Build history of the part. All positions in model axes, mm. Face numbers are marked on the shaded views. A direction names the side the tool comes from. Give positions to 0.01 mm unless a question says otherwise; leave off trailing zeros. Loops run counter-clockwise (first coordinate to the right, second up) from the corner with the lowest first, then second, coordinate; pieces in that order, holes last. Notation, with made-up numbers: (66.25, 15) - (79.25, 15) arc R6 cw to (79.25, 24) - close; hole circle Ø10 at (5.5, -30). An arc over 180 degrees is marked (long way). Return JSON: item names as keys, results as strings. Group by question number.
1) Drop flat-ended pins along their axis: pin 1 (4 mm diameter, centred on x = -3.5, y = 48, fed in from -Z); pin 2 (19 mm diameter, centred on y = 18.5, z = 6.5, fed in from -X); pin 3 (8 mm diameter, centred on x = 29.5, z = 0.5, fed in from -Y). Give the stop position or say it passes through.
2) Slice it at B-B (y = -7). List the corners of the cut face in (x, z), and give its area (3 significant figures).
3) Mould opens along Z. For the marked faces 6, 7 and 8 say: released by +Z, released by -Z, zero draft, split by the parting line, or undercut.
4) Slice it at C-C (x = 12.5). List the corners of the cut face in (y, z).
5) Slice it at D-D (y = 34). List the corners of the cut face in (x, z).
6) 3-axis set-ups, long thin cutter, end or side, ignore diameter. For the marked faces 1, 2, 3, 4 and 5: which of +Z, -Z, +X, -X, +Y, -Y reach the whole face in a straight line?
7) Drill centre lines: probe 1 along Y at (x, z) = (-7, 0); probe 2 along Z at (x, y) = (4.5, 10.5); probe 3 along X at (y, z) = (49, 19). Where is each one in solid material? Low to high. Write a range as from..to.
8) Slice it at A-A (z = 10). List the corners of the cut face in (x, y).
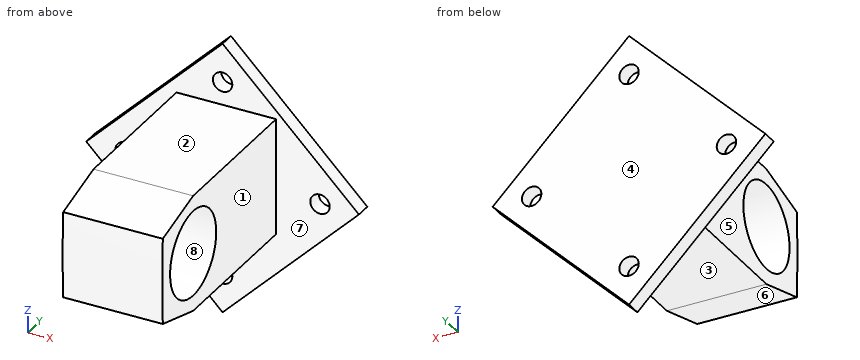
```python
from build123d import *

# Parameters (mm, degrees)
SKETCH1_W           = 32.512
SKETCH1_H           = 38.1
BOSS_EXTRUDE1_DEPTH = 50.292
BOSS_EXTRUDE2_DEPTH = 32.512
SKETCH3_R           = 13.9871704
CUT_EXTRUDE1_DEPTH  = 127
BOSS_EXTRUDE3_DEPTH = 5.08
SKETCH5_R           = 3.175
CUT_EXTRUDE2_DEPTH  = 101.256951791


with BuildPart() as part:
    # Sketch1 → Boss-Extrude1 (new body)
    with BuildSketch(Plane(origin=(0, 0, 0), x_dir=(1, 0, 0), z_dir=(0, 1, 0))):
        Rectangle(SKETCH1_W, SKETCH1_H)
    extrude(amount=BOSS_EXTRUDE1_DEPTH)

    # Sketch2 → Boss-Extrude2 (add)
    with BuildSketch(Plane(origin=(16.256, 0, 0), x_dir=(0, 0, -1), z_dir=(1, 0, 0))):
        with BuildLine():
            Line((-19.05, 0), (-14.119497191, -18.400886991))
            ThreePointArc((-14.119497191, -18.400886991), (0, -18.733351542), (14.119497191, -18.400886991))
            Line((14.119497191, -18.400886991), (19.05, 0))
            Line((19.05, 0), (-19.05, 0))
        make_face()
    extrude(amount=-BOSS_EXTRUDE2_DEPTH)

    # Sketch3 → Cut-Extrude1 (cut)
    with BuildSketch(Plane(origin=(16.256, 0, 0), x_dir=(0, 0, -1), z_dir=(1, 0, 0))):
        Circle(SKETCH3_R)
    extrude(amount=-CUT_EXTRUDE1_DEPTH, mode=Mode.SUBTRACT)

    # Sketch4 → Boss-Extrude3 (add)
    with BuildSketch(Plane(origin=(0, 50.292, 0), x_dir=(1, 0, 0), z_dir=(0, 1, 0))):
        Polygon((-1.207933769, -39.277381208), (-45.702074629, 5.216759653), (-1.207933769, 49.710900513), (43.286207092, 5.216759653), align=None)
    extrude(amount=BOSS_EXTRUDE3_DEPTH)

    # Sketch5 → Cut-Extrude2 (cut, through all)
    with BuildSketch(Plane(origin=(0, 55.372, 0), x_dir=(1, 0, 0), z_dir=(0, 1, 0))):
        with Locations(Location((30.586207092, 5.216759653, 0), (0, 0, 270))):
            Circle(SKETCH5_R)
        with Locations(Location((-1.207933769, -26.577381208, 0), (0, 0, 270))):
            Circle(SKETCH5_R)
        with Locations(Location((-1.207933769, 37.010900513, 0), (0, 0, 90))):
            Circle(SKETCH5_R)
        with Locations(Location((-33.002074629, 5.216759653, 0), (0, 0, 90))):
            Circle(SKETCH5_R)
    extrude(amount=-CUT_EXTRUDE2_DEPTH, mode=Mode.SUBTRACT)


solid = part.part
```
Results:
{
 "1": {"pin 1": "z = -19.05", "pin 2": "x = -16.26", "pin 3": "y = 50.29"},
 "2": {"outline": "(-16.26, -17.17) - (16.26, -17.17) - (16.26, -12.11) - (-16.26, -12.11) - close; (-16.26, 12.11) - (16.26, 12.11) - (16.26, 17.17) - (-16.26, 17.17) - close", "area": "329 mm2"},
 "3": {"face 6": "released by -Z", "face 7": "zero draft", "face 8": "undercut"},
 "4": {"outline": "(-18.4, -14.12) - (0, -19.05) - (50.29, -19.05) - (50.29, -36) - (55.37, -36) - (55.37, 25.57) - (50.29, 25.57) - (50.29, 19.05) - (0, 19.05) - (-18.4, 14.12) arc R299.99 ccw to start; hole circle Ø27.97 at (0, 0)"},
 "5": {"outline": "(-16.26, -19.05) - (16.26, -19.05) - (16.26, 19.05) - (-16.26, 19.05) - close"},
 "6": {"face 1": "+Z, -Z, +X, -Y", "face 2": "+Z, +X, -X, -Y", "face 3": "-Z, +X, -X, -Y", "face 4": "+Z, -Z, +X, -X, +Y", "face 5": "+Z, -Z, -X, -Y"},
 "7": {"probe 1": "-18.73..-13.99, 13.99..55.37", "probe 2": "-19.05..-9.24, 9.24..19.05", "probe 3": "-16.26..16.26"},
 "8": {"outline": "(-30.49, 50.29) - (-16.26, 50.29) - (-16.26, 9.78) - (16.26, 9.78) - (16.26, 50.29) - (28.07, 50.29) - (28.07, 55.37) - (-30.49, 55.37) - close; (-16.26, -18.57) - (16.26, -18.57) - (16.26, -9.78) - (-16.26, -9.78) - close"}
}
